Source: CAD feature listing. Evaluate the final solid. Frame: model axes, mm. A direction names the side the tool comes from. Give positions to 0.01 mm unless a question says otherwise; leave off trailing zeros. Loops run counter-clockwise (first coordinate to the right, second up) from the corner with the lowest first, then second, coordinate; pieces in that order, holes last.
```python
from build123d import *

# Parameters (mm, degrees)
CROQUIS4_R              = 2.75
SALIENTE_EXTRUIR3_DEPTH = 3
CHAFL_N2_SIZE           = 0.3
CROQUIS6_R              = 1.5
SALIENTE_EXTRUIR4_DEPTH = 5


with BuildPart() as part:
    # Croquis4 → Saliente-Extruir3 (new body)
    with BuildSketch(Plane(origin=(0, 0, 0), x_dir=(1, 0, 0), z_dir=(0, 1, 0))):
        with Locations(Location((0, 0, 0), (0, 0, 270))):
            Circle(CROQUIS4_R)
        Polygon((0, 1.25), (-1.082531755, 0.625), (-1.082531755, -0.625), (0, -1.25), (1.082531755, -0.625), (1.082531755, 0.625), align=None, mode=Mode.SUBTRACT)
    extrude(amount=SALIENTE_EXTRUIR3_DEPTH)

    # Chafl_n2
    chafl_n2_edges = [part.edges().sort_by_distance(p)[0] for p in [
        (0, 3, -2.75),
    ]]
    chamfer(chafl_n2_edges, length=CHAFL_N2_SIZE)

    # Croquis5 → Revoluci_n2 (revolve)
    with BuildSketch(Plane.XY, mode=Mode.PRIVATE) as revoluci_n2_sk:
        Polygon((0, 0), (0, 0.778312164), (1.25, 1.5), (2.75, 1.5), (2.75, 0), align=None)
    revolve(revoluci_n2_sk.sketch.rotate(Axis((0, 0, 0), (0, 1, 0)), 180), axis=Axis((0, 0, 0), (0, 1, 0)))

    # Croquis6 → Saliente-Extruir4 (add)
    with BuildSketch(Plane.XZ):
        with Locations(Location((0, 0, 0), (0, 0, 90))):
            Circle(CROQUIS6_R)
    extrude(amount=SALIENTE_EXTRUIR4_DEPTH)


solid = part.part
```
(1) First-contact query: pin 1 (1 mm diameter, centred on x = -0.5, y = -1.5, fed in from +Z); pin 2 (2 mm diameter, centred on x = -0.5, y = -3.5, fed in from -Z); pin 3 (2 mm diameter, centred on x = -1.5, y = -3.5, fed in from -Z). Flat tips, straight axial feed; report the tip coordinate or a pass-through.
A:
pin 1: stops at z = 1.5
pin 2: stops at z = -1.5
pin 3: stops at z = -1.41
(2) Reachability of faces 4 (the cylindrical face through (-0.45, -2.46, 1.43)), 5 (the flat face through (0, -5, 0)), 6 (the flat face through (1.083, 2, 0)) from +Z, -Z, +X, -X, +Y, -Y: full face, straight path, thin tool, end or side. Return the list, or none.
A:
face 4: -Y
face 5: +Z, -Z, +X, -X, -Y
face 6: +Y
(3) Section B-B, the plane y = 0.5. Return the cut outline in (x, z), then the cut area to 3 significant figures.
A:
outline: circle Ø5.5 at (0, 0)
area: 23.8 mm2
(4) Ray query, line 1 along Z through (x, y) = (1.25, 2.25); line 2 along X through (y, z) = (-1.5, -0.05); line 3 along Y through (x, z) = (1.7, -1.25). Return the intervals inside material, ascending.
A:
line 1: z = -2.45 to 2.45
line 2: x = -1.5 to 1.5
line 3: y = 0 to 3
(5) Mould query, pull axis Z, two halves, no side actions, for faces 1 (the flat face through (0.534, 2.19, 0.942)), 2 (the flat face through (-1, 3, 1)), 3 (the cylindrical face through (-2.685, 1.331, -0.596)). Classes: pulls with the +Z half, pulls with the -Z half, needs draft (parallel to the pull), parting line crosses it, or undercut.
A:
face 1: undercut
face 2: needs draft
face 3: parting line crosses it
(6) Section A-A, the plane y = -1. Return the cut outline in (x, z).
A:
outline: circle Ø3 at (0, 0)
